Geometry check sheet. Reference: the model listing, model coordinates, mm. A direction names the side the tool comes from. Round coordinates to 2 decimals unless told otherwise and drop trailing zeros. Write each loop counter-clockwise with the first axis right and the second up, starting at its lowest first coordinate (ties: lowest second). Pieces come first, ordered by that corner, then holes. Notation, with made-up numbers: (5.5, -36) -> (27.5, -36) arc R11 cw to (27.5, -27) -> close; hole circle Ø7 at (25.25, -35.5). An arc over 180 degrees is marked (long way). Use a Markdown table: item, result.
```python
from build123d import *

# Parameters (mm, degrees)
SKETCH_1_R              = 2.75
EXTRUDE_1_DEPTH         = 2
SKETCH_2_R              = 1.05
EXTRUDE_13689_DEPTH     = 3
SKETCH_3_W              = 3
SKETCH_3_H              = 36
SKETCH_3_W_2            = 3.45
EXTRUDE_14140_DEPTH     = 20
CUT_EXTRUDE_14477_REACH = 157.33
SKETCH_5_R              = 1.05
SKETCH_6_R              = 1.245588001
EXTRUDE_15246_DEPTH     = 3
FILLET_1_R              = 1


with BuildPart() as part:
    # 草图1 → 凸台-拉伸1 (new body)
    with BuildSketch(Plane.XY):
        with BuildLine():
            Line((-31.232935168, 137.582300402), (-39.033457742, 137.582300402))
            ThreePointArc((-39.033457742, 137.582300402), (-40.802630101, 137.2588407), (-42.342900075, 136.330312067))
            Line((-42.342900075, 136.330312067), (-44.480254451, 134.443057788))
            ThreePointArc((-44.480254451, 134.443057788), (-45.728619247, 132.750865708), (-46.170812117, 130.695046123))
            Line((-46.170812117, 130.695046123), (-46.170812117, 97.620783931))
            ThreePointArc((-46.170812117, 97.620783931), (-45.830898888, 96.66237235), (-44.963075466, 96.132300402))
            Line((-44.963075466, 96.132300402), (-39.335406059, 94.947479812))
            Line((-39.335406059, 94.947479812), (-36.200029499, 92.942583722))
            Line((-36.200029499, 92.942583722), (-36.200029499, 89.608050871))
            Line((-36.200029499, 89.608050871), (-19.688242157, 78.763336754))
            Line((-19.688242157, 78.763336754), (-14.532154357, 78.763336754))
            Line((-14.532154357, 78.763336754), (-9.532154357, 83.763336754))
            Line((-9.532154357, 83.763336754), (9.532154357, 83.763336754))
            Line((9.532154357, 83.763336754), (14.532154357, 78.763336754))
            Line((14.532154357, 78.763336754), (19.688242157, 78.763336754))
            Line((19.688242157, 78.763336754), (36.200029499, 89.608050871))
            Line((36.200029499, 89.608050871), (36.200029499, 92.942583722))
            Line((36.200029499, 92.942583722), (39.335406059, 94.947479812))
            Line((39.335406059, 94.947479812), (44.963075466, 96.132300402))
            ThreePointArc((44.963075466, 96.132300402), (45.830898888, 96.66237235), (46.170812117, 97.620783931))
            Line((46.170812117, 97.620783931), (46.170812117, 130.695046123))
            ThreePointArc((46.170812117, 130.695046123), (45.728619247, 132.750865708), (44.480254451, 134.443057788))
            Line((44.480254451, 134.443057788), (42.342900075, 136.330312067))
            ThreePointArc((42.342900075, 136.330312067), (40.802630101, 137.2588407), (39.033457742, 137.582300402))
            Line((39.033457742, 137.582300402), (31.232935168, 137.582300402))
            ThreePointArc((31.232935168, 137.582300402), (32.726681953, 116.126426191), (31.232935168, 94.67055198))
            Line((31.232935168, 94.67055198), (-31.232935168, 94.67055198))
            ThreePointArc((-31.232935168, 94.67055198), (-32.726681953, 116.126426191), (-31.232935168, 137.582300402))
        make_face()
        with Locations((39.335406059, 129.082300402)):
            Circle(SKETCH_1_R, mode=Mode.SUBTRACT)
        with Locations((39.335406059, 104.082300402)):
            Circle(SKETCH_1_R, mode=Mode.SUBTRACT)
        with Locations((17.23796389, 84.763336754)):
            Circle(SKETCH_1_R, mode=Mode.SUBTRACT)
        with Locations(Location((-17.23796389, 84.763336754, 0), (0, 0, 180))):
            Circle(SKETCH_1_R, mode=Mode.SUBTRACT)
        with Locations(Location((-39.335406059, 104.082300402, 0), (0, 0, 180))):
            Circle(SKETCH_1_R, mode=Mode.SUBTRACT)
        with Locations(Location((-39.335406059, 129.082300402, 0), (0, 0, 180))):
            Circle(SKETCH_1_R, mode=Mode.SUBTRACT)
    extrude(amount=EXTRUDE_1_DEPTH)

    # 草图2 → Extrude 13689 (add)
    with BuildSketch(Plane(origin=(0, 94.67055198, 0), x_dir=(1, 0, 0), z_dir=(0, 1, 0))):
        Polygon((12.371090345, 0), (19.75, 0), (19.75, -36), (12.7, -36), (12.7, -8.95), (-12.7, -8.95), (-12.7, -36), (-25.75, -36), (-25.75, 0), (-12.371090345, 0), align=None)
        with Locations(Location((14.75, -10, 0), (0, 0, 270))):
            Circle(SKETCH_2_R, mode=Mode.SUBTRACT)
        with Locations(Location((-14.75, -10, 0), (0, 0, 90))):
            Circle(SKETCH_2_R, mode=Mode.SUBTRACT)
        with Locations(Location((-14.75, -22, 0), (0, 0, 270))):
            Circle(SKETCH_2_R, mode=Mode.SUBTRACT)
        with Locations(Location((14.75, -22, 0), (0, 0, 90))):
            Circle(SKETCH_2_R, mode=Mode.SUBTRACT)
    extrude(amount=EXTRUDE_13689_DEPTH)

    # 草图3 → Extrude 14140 (add)
    with BuildSketch(Plane(origin=(0, 97.67055198, 0), x_dir=(1, 0, 0), z_dir=(0, 1, 0))):
        with Locations((-24.25, -18)):
            Rectangle(SKETCH_3_W, SKETCH_3_H)
        with Locations((18.025, -18)):
            Rectangle(SKETCH_3_W_2, SKETCH_3_H)
    extrude(amount=EXTRUDE_14140_DEPTH)

    # 草图5 → Cut-Extrude 14477 (cut, up to next)
    with BuildSketch(Plane.ZY.offset(-16.3), mode=Mode.PRIVATE) as cut_extrude_14477_sk1:
        with Locations((12, 102.17055198)):
            Circle(SKETCH_5_R)
    cut_extrude_14477_tool1 = extrude(cut_extrude_14477_sk1.sketch, amount=-CUT_EXTRUDE_14477_REACH, mode=Mode.PRIVATE) & part.part
    # 草图5 → Cut-Extrude 14477 (cut, up to next)
    with BuildSketch(Plane.ZY.offset(-16.3), mode=Mode.PRIVATE) as cut_extrude_14477_sk2:
        with Locations((12, 112.17055198)):
            Circle(SKETCH_5_R)
    cut_extrude_14477_tool2 = extrude(cut_extrude_14477_sk2.sketch, amount=-CUT_EXTRUDE_14477_REACH, mode=Mode.PRIVATE) & part.part
    # 草图5 → Cut-Extrude 14477 (cut, up to next)
    with BuildSketch(Plane.ZY.offset(-16.3), mode=Mode.PRIVATE) as cut_extrude_14477_sk3:
        with BuildLine():
            Line((7.5, 112.298234054), (7.5, 110.096723462))
            Line((7.5, 110.096723462), (30.937767474, 110.096723462))
            Line((30.937767474, 110.096723462), (30.937767474, 107.500731647))
            Line((30.937767474, 107.500731647), (7.5, 107.500731647))
            Line((7.5, 107.500731647), (7.5, 103.107695613))
            ThreePointArc((7.5, 103.107695613), (6, 101.607695613), (4.5, 103.107695613))
            Line((4.5, 103.107695613), (4.5, 112.298234054))
            ThreePointArc((4.5, 112.298234054), (6, 113.798234054), (7.5, 112.298234054))
        make_face()
    cut_extrude_14477_tool3 = extrude(cut_extrude_14477_sk3.sketch, amount=-CUT_EXTRUDE_14477_REACH, mode=Mode.PRIVATE) & part.part
    add(cut_extrude_14477_tool1.solids().sort_by_distance((16.3, 102.170552, 12))[0], mode=Mode.SUBTRACT)
    add(cut_extrude_14477_tool2.solids().sort_by_distance((16.3, 112.170552, 12))[0], mode=Mode.SUBTRACT)
    add(cut_extrude_14477_tool3.solids().sort_by_distance((16.3, 108.401203, 14.423289))[0], mode=Mode.SUBTRACT)

    # 草图6 → Extrude 15246 (add)
    with BuildSketch(Plane(origin=(0, 0, 0), x_dir=(-1, 0, 0), z_dir=(0, 0, -1))):
        Polygon((-16.3, 117.67055198), (-9.937167199, 117.67055198), (-7.741837129, 115.189840313), (14.191837129, 115.189840313), (16.387167199, 117.67055198), (22.75, 117.67055198), (22.75, 97.67055198), (-16.3, 97.67055198), align=None)
        with Locations((-12.775, 114.69834671)):
            Circle(SKETCH_6_R, mode=Mode.SUBTRACT)
        with Locations((19.225, 114.69834671)):
            Circle(SKETCH_6_R, mode=Mode.SUBTRACT)
        with Locations((-12.775, 102.69834671)):
            Circle(SKETCH_6_R, mode=Mode.SUBTRACT)
        with Locations((19.225, 102.69834671)):
            Circle(SKETCH_6_R, mode=Mode.SUBTRACT)
        with BuildLine():
            Line((-3.280276477, 101.336740903), (9.730276477, 101.336740903))
            ThreePointArc((9.730276477, 101.336740903), (11.230276477, 99.836740903), (9.730276477, 98.336740903))
            Line((9.730276477, 98.336740903), (-3.280276477, 98.336740903))
            ThreePointArc((-3.280276477, 98.336740903), (-4.780276477, 99.836740903), (-3.280276477, 101.336740903))
        make_face(mode=Mode.SUBTRACT)
    extrude(amount=-EXTRUDE_15246_DEPTH)

    # 圆角1
    fillet_1_edges = [part.edges().sort_by_distance(p)[0] for p in [
        (19.75, 94.67055198, 1),
        (-25.75, 94.67055198, 1),
        (-12.7, 96.17055198, 8.95),
        (12.7, 96.17055198, 8.95),
        (18.025, 110.096723462, 7.5),
        (18.025, 110.096723462, 30.937767474),
        (18.025, 107.500731647, 30.937767474),
        (18.025, 107.500731647, 7.5),
        (-31.232935168, 94.67055198, 1),
        (31.232935168, 94.67055198, 1),
    ]]
    fillet(fillet_1_edges, radius=FILLET_1_R)


solid = part.part
```
(1) Section check B-B on z = 6. Record the cut outline in (x, y), plus the area to 3 significant figures.
A:
| item | result |
|---|---|
| outline | (-25.75, 94.67) -> (19.75, 94.67) -> (19.75, 101.61) -> (16.3, 101.61) -> (16.3, 97.67) -> (-22.75, 97.67) -> (-22.75, 117.67) -> (-25.75, 117.67) -> close; (16.3, 113.8) -> (19.75, 113.8) -> (19.75, 117.67) -> (16.3, 117.67) -> close |
| area | 223 mm2 |
(2) Section check A-A on z = 22. Record the cut outline in (x, y), plus the area to 3 significant figures.
A:
| item | result |
|---|---|
| outline | (-25.75, 94.67) -> (-15.8, 94.67) -> (-15.8, 97.67) -> (-22.75, 97.67) -> (-22.75, 117.67) -> (-25.75, 117.67) -> close; (-13.7, 94.67) -> (-12.7, 94.67) -> (-12.7, 97.67) -> (-13.7, 97.67) -> close; (12.7, 94.67) -> (13.7, 94.67) -> (13.7, 97.67) -> (12.7, 97.67) -> close; (15.8, 94.67) -> (19.75, 94.67) -> (19.75, 107.5) -> (16.3, 107.5) -> (16.3, 97.67) -> (15.8, 97.67) -> close; (16.3, 110.1) -> (19.75, 110.1) -> (19.75, 117.67) -> (16.3, 117.67) -> close |
| area | 168 mm2 |
(3) Thickness scan on line 1 (Y direction, x = 18.15, z = 12); line 2 (X direction, y = 96, z = 10); line 3 (Z direction, x = 14, y = 95). Record the ranges inside material, lowest first.
A:
| item | result |
|---|---|
| line 1 | y = 94.67 to 101.12, 103.22 to 107.5, 110.1 to 111.12, 113.22 to 117.67 |
| line 2 | x = -25.75 to -15.8, -13.7 to -12.7, 12.7 to 13.7, 15.8 to 19.75 |
| line 3 | z = 0 to 9.27, 10.73 to 21.27, 22.73 to 36 |
(4) Gauge pin test, flat ends, axial feed: pin 1 Ø4 at (y, z) = (112, 28) entering from +X; pin 2 Ø1.5 at (x, z) = (-12, 19) entering from -Y; pin 3 Ø2 at (x, z) = (25, 0.5) entering from +Y. Record the tip position at first contact, or that the pin passes through.
A:
| item | result |
|---|---|
| pin 1 | stops at x = 19.75 |
| pin 2 | stops at y = 94.67 |
| pin 3 | stops at y = 94.67 |
(5) Release check for a two-part mould opening along X. For faces 6 (the face through (-11.23, 99.87, 1.48)), 7 (the face through (-43.397, 135.4, 0.986)), 8 (the face through (-3, 115.19, 1)), 9 (the face through (45.741, 132.724, 0.986)) record: +X half, -X half, draft (parallel to the pull), parting line (faces both ways), or undercut.
A:
| item | result |
|---|---|
| face 6 | undercut |
| face 7 | -X half |
| face 8 | undercut |
| face 9 | +X half |
(6) Section check D-D on y = 100. Record the cut outline in (x, z), plus the area to 3 significant figures.
A:
| item | result |
|---|---|
| outline | (-46.17, 0) -> (-31.88, 0) -> (-31.88, 2) -> (-46.17, 2) -> close; (-25.75, 0) -> (-11.22, 0) -> (-11.22, 3) -> (-22.75, 3) -> (-22.75, 36) -> (-25.75, 36) -> close; (4.77, 0) -> (19.75, 0) -> (19.75, 36) -> (16.3, 36) -> (16.3, 3) -> (4.77, 3) -> close; (31.88, 0) -> (46.17, 0) -> (46.17, 2) -> (31.88, 2) -> close |
| area | 359 mm2 |
(7) Access from +Z, -Z, +X, -X, +Y, -Y to the whole of each face (thin tool, end or side, straight path). Record for faces 1 (the face through (-32.727, 116.269, 0.986)), 2 (the face through (-7, 97.671, 8)), 3 (the face through (14.35, 96.15, 10.97)), 4 (the face through (11.997, 81.298, 0.986)), 5 (the face through (18, 105, 7.5)).
A:
| item | result |
|---|---|
| face 1 | +Z, -Z |
| face 2 | +Z, +Y |
| face 3 | +Y, -Y |
| face 4 | +Z, -Z, -Y |
| face 5 | +X |
(8) Section check C-C on y = 124.5. Record the cut outline in (x, z), plus the area to 3 significant figures.
A:
| item | result |
|---|---|
| outline | (-46.17, 0) -> (-32.5, 0) -> (-32.5, 2) -> (-46.17, 2) -> close; (32.5, 0) -> (46.17, 0) -> (46.17, 2) -> (32.5, 2) -> close |
| area | 54.7 mm2 |
